Read the model definition and answer for the solid it produces. Units are mm, in the model's axes. Round coordinates to 2 decimals unless told otherwise and drop trailing zeros. Order: outer loops, then holes, each group sorted by start corner. A loop starts at its lowest first (then second) coordinate and runs counter-clockwise, first axis right, second up. Notation, with made-up numbers: (-18.5, 33.25) - (-4.5, 33.25) arc R32 cw to (-4.5, 68.25) - close; hole circle Ø6 at (-11.75, 74.5). An arc over 180 degrees is marked (long way). Put each result on its own line as item: value. Start each with the question number.
Q1. Find the intervals of material crossed by line 1 along X through (y, z) = (1.85, 0); line 2 along Z through (x, y) = (-45, 2.1); line 3 along Z through (x, y) = (-68, 0.95), in increasing order. Write a range as from..to.
Q2. Section B-B on z = 0 is taken. Give the vertices of the cut face in (x, y).
Q3. Section A-A on x = -38 is taken. Give the vertices of the cut face in (y, z), then the cut area to 3 significant figures.
Q4. Each of these flat-tipped pins is pushed along its axis until it touches: pin 1 Ø1.5 at (x, y) = (-61.5, 1) entering from +Z; pin 2 Ø0.9 at (y, z) = (1.5, 26) entering from +X; pin 3 Ø1.5 at (x, y) = (-60, 2.5) entering from +Z; pin 4 Ø2.5 at (x, z) = (0, 0) entering from -Y. Where does it stop, or does it pass through?
Q5. Section D-D on x = -71.5 is taken. Give the vertices of the cut face in (y, z), then the cut area to 3 significant figures.
Q6. Section C-C on y = 2.5 is taken. Give the vertices of the cut face in (x, z).
from build123d import *

# Parameters (mm, degrees)
SKETCH_1_R      = 1.5
EXTRUDE_1_DEPTH = 3
FILLET_5_R      = 15


with BuildPart() as part:
    # 草图1 → 凸台-拉伸1 (new body)
    with BuildSketch(Plane(origin=(0, 0, 0), x_dir=(1, 0, 0), z_dir=(0, 1, 0))):
        with BuildLine():
            Line((0, 5), (-60, 5))
            Line((-60, 5), (-82.371742522, -23.015711498))
            Line((-82.371742522, -23.015711498), (-87.879028911, -23.015711498))
            Line((-87.879028911, -23.015711498), (-87.879028911, -28.015711498))
            Line((-87.879028911, -28.015711498), (-62.879028911, -28.015711498))
            Line((-62.879028911, -28.015711498), (-62.879028911, -23.015711498))
            Line((-62.879028911, -23.015711498), (-68.3863153, -23.015711498))
            Line((-68.3863153, -23.015711498), (-54, -5))
            Line((-54, -5), (0, -5))
            ThreePointArc((0, -5), (5, 0), (0, 5))
        make_face()
        with Locations(Location((0, 0, 0), (0, 0, 270))):
            Circle(SKETCH_1_R, mode=Mode.SUBTRACT)
        with Locations(Location((-38, 0, 0), (0, 0, 270))):
            Circle(SKETCH_1_R, mode=Mode.SUBTRACT)
    extrude(amount=EXTRUDE_1_DEPTH)

    # 圆角5
    fillet_5_edges = [part.edges().sort_by_distance(p)[0] for p in [
        (-54, 1.5, 5),
    ]]
    fillet(fillet_5_edges, radius=FILLET_5_R)


solid = part.part
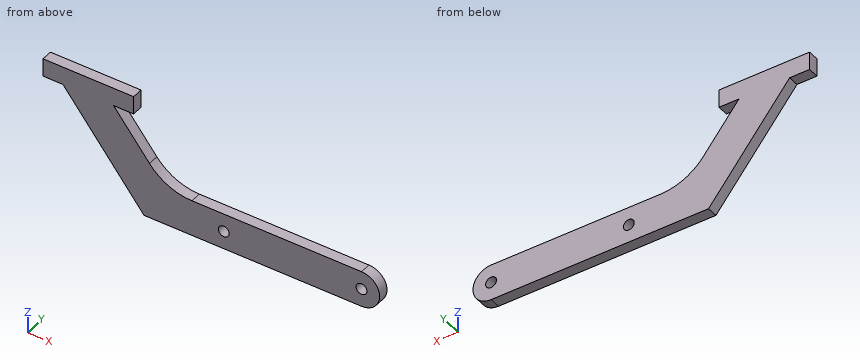
Findings:
1. line 1: -63.99..-39.5, -36.5..-1.5, 1.5..5
1. line 2: -5..5
1. line 3: 5.02..22.53, 23.02..28.02
2. outline: (-63.99, 0) - (-39.5, 0) - (-39.5, 3) - (-63.99, 3) - close; (-36.5, 0) - (-1.5, 0) - (-1.5, 3) - (-36.5, 3) - close; (1.5, 0) - (5, 0) - (5, 3) - (1.5, 3) - close
3. outline: (0, -5) - (3, -5) - (3, -1.5) - (0, -1.5) - close; (0, 1.5) - (3, 1.5) - (3, 5) - (0, 5) - close
3. area: 21.0 mm2
4. pin 1: z = 15.33
4. pin 2: x = -62.88
4. pin 3: z = 13.45
4. pin 4: through
5. outline: (0, 9.4) - (3, 9.4) - (3, 28.02) - (0, 28.02) - close
5. area: 55.8 mm2
6. outline: (-87.88, 23.02) - (-82.37, 23.02) - (-60, -5) - (0, -5) arc R5 ccw to (0, 5) - (-46.78, 5) arc R15 cw to (-58.5, 10.64) - (-68.39, 23.02) - (-62.88, 23.02) - (-62.88, 28.02) - (-87.88, 28.02) - close; hole circle Ø3 at (-38, 0); hole circle Ø3 at (0, 0)
